Geometry: see drawing. Coordinates: mm, zero at the bounding-box minimum. Round coordinates to 2 decimals unless told otherwise and drop trailing zeros. Loops run counter-clockwise (first coordinate to the right, second up) from the corner with the lowest first, then second, coordinate; pieces in that order, holes last. Notation, with made-up numbers: (-7.75, -37.5) - (46.25, -37.5) arc R25 ccw to (46.25, -0.5) - close; hole circle Ø1 at (6, 4.5). An arc over 180 degrees is marked (long way). Write item = value, one per line. Start each with the question number.
Item 1: Draft query along Y for the marked faces 1, 2 and 3. Return one class per face: pulls with the +Y half, pulls with the -Y half, needs draft (parallel to the pull), parting line crosses it, or undercut.
Item 2: Section A-A (y = 7). Return loops of the section in (x, z).
Item 3: First-contact query: pin 1 (5 mm diameter, centred on x = 5, z = 3, fed in from -Y); pin 2 (3 mm diameter, centred on y = 8, z = 3, fed in from +X); pin 3 (5 mm diameter, centred on x = 5, z = 5.5, fed in from -Y). Flat tips, straight axial feed; report the tip coordinate or a pass-through.
Item 4: Section C-C (z = 4.25). Return loops of the section in (x, y).
Item 5: Line query: line 1 (Y direction, x = 7, z = 3.75); line 2 (X direction, y = 8.25, z = 0.5); line 3 (X direction, y = 2.5, z = 6). Output: solid intervals per line, ascending. Write a range as from..to.
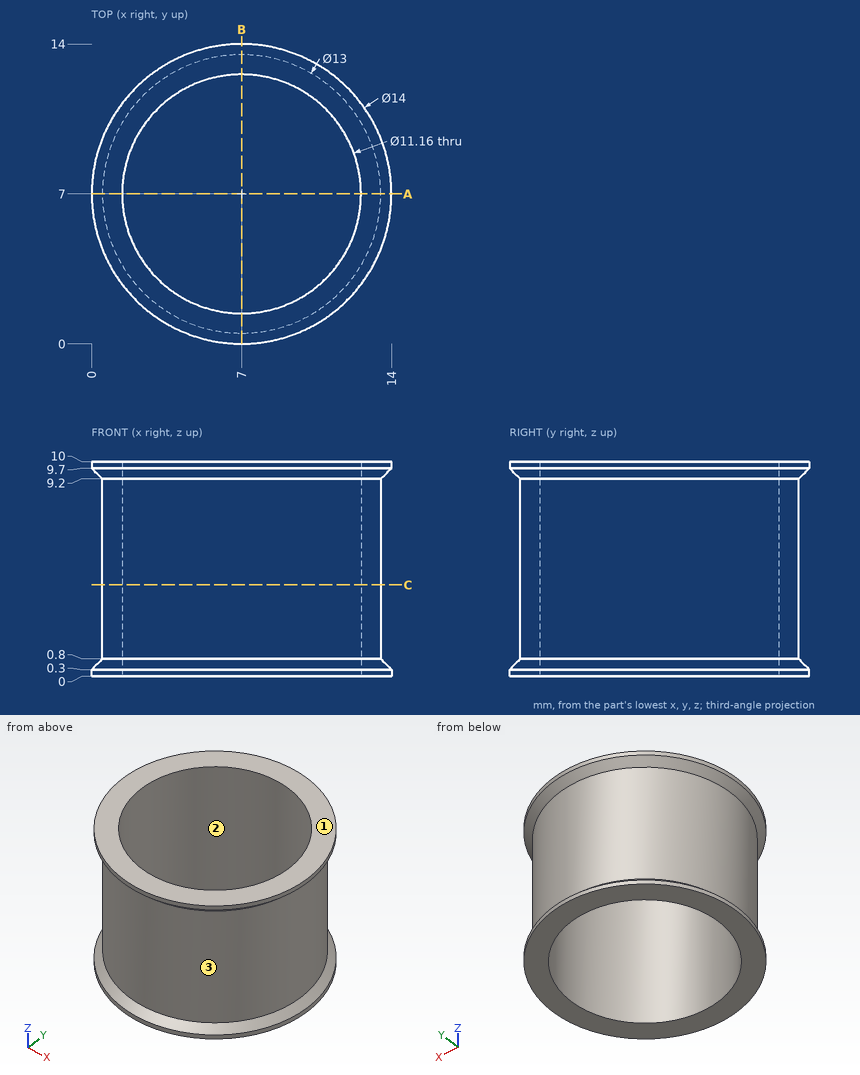
Taken from the geometry:
q1.face_1 = needs draft
q1.face_2 = undercut
q1.face_3 = parting line crosses it
q2.outline = (0, 0) - (1.42, 0) - (1.42, 10) - (0, 10) - (0, 9.7) - (0.5, 9.2) - (0.5, 0.8) - (0, 0.3) - close; (12.58, 0) - (14, 0) - (14, 0.3) - (13.5, 0.8) - (13.5, 9.2) - (14, 9.7) - (14, 10) - (12.58, 10) - close
q3.pin_1 = 0.42
q3.pin_2 = 13.5
q3.pin_3 = 0.5
q4.outline = circle Ø13 at (7, 7); hole circle Ø11.16 at (7, 7)
q5.line_1 = 0.5..1.42, 12.58..13.5
q5.line_2 = 0.32..1.56, 12.44..13.68
q5.line_3 = 2.31..3.7, 10.3..11.69
